CAD build for the part. Positions are in the model's coordinates, mm. A direction names the side the tool comes from. Round coordinates to 2 decimals unless told otherwise and drop trailing zeros. Loops run counter-clockwise (first coordinate to the right, second up) from the corner with the lowest first, then second, coordinate; pieces in that order, holes last. Notation, with made-up numbers: M 54.5,88.25 L 69.5,88.25 A13 ccw 69.5,93.25 Z; hole C 49,-23 d7. An arc over 180 degrees is marked long. Use a Markdown table: item, result. Add a question column.
(1) Band-saw the part on C-C, the plane x = 0. Write the cut outline in (y, z), and give its area (3 significant figures).
(2) Band-saw the part on B-B, the plane z = -22.5. Write the cut outline in (x, y), and give its area (4 significant figures).
(3) Band-saw the part on A-A, the plane y = 42. Write the cut outline in (x, z), and give its area (3 significant figures).
(4) Band-saw the part on D-D, the plane z = 37. Write the cut outline in (x, y), and give its area (3 significant figures).
(5) Flat gauge pins, fed straight in: P1, Ø1, axis at x = -55.5, z = -54, coming from the -Y side; P2, Ø10, axis at x = 7, z = 30.5, coming from the +Y side; P3, Ø2.5, axis at x = 34.5, y = 20.4, coming from the -Z side; P4, Ø6, axis at x = 43.5, y = 22.5, coming from the -Z side. Where does each tip first touch, or does it go through?
(6) Which spindle directions (+Z, -Z, +X, -X, +Y, -Y) get a long thin tool onto all of the face, cutting with end or side? Do faces 5 (the face through (6, 18, 52.5)), 6 (the face through (47.263, 26.302, 53.486)). Say none if no direction does.
(7) Two-plate mould, pull along Z, no slides. Class faces 1 (the face through (-79.398, 21.336, -53.514)), 2 (the face through (6, 18, 54.5)), 3 (the face through (9, 14, -54.5)), 4 (the face through (-2, 0, -1)): released by +Z, released by -Z, zero draft, split by the parting line, or undercut.
(8) Wall check: L1, parallel to Z at x = 75, y = 5; L2, parallel to Y at x = 43, z = 53; L3, parallel to Y at x = 43.5, z = -53.2. Give the ranges that are in metal, low to high.
from build123d import *

# Parameters (mm, degrees)
SKETCH3_W                       = 250
SKETCH3_H                       = 105
BASE_FLANGE1_DEPTH              = 2
EDGE_FLANGE1_STRIP_W            = 10
EDGE_FLANGE1_STRIP_H            = 2
EDGE_FLANGE1_STRIP_CUT_DEPTH    = 217
EDGE_FLANGE1_RELIEF_W           = 11
EDGE_FLANGE1_RELIEF_H           = 1
EDGE_FLANGE1_RELIEF_CUT_DEPTH   = 2
EDGE_FLANGE1_STRIP_2_W          = 10
EDGE_FLANGE1_STRIP_2_H          = 2
EDGE_FLANGE1_STRIP_CUT_2_DEPTH  = 217
EDGE_FLANGE1_RELIEF_2_W         = 11
EDGE_FLANGE1_RELIEF_2_H         = 1
EDGE_FLANGE1_RELIEF_CUT_2_DEPTH = 2
EDGE_FLANGE1_DEPTH              = 217
EDGE_FLANGE1_START              = 2
EDGE_FLANGE1_PROFILE_R          = 5
EDGE_FLANGE1_FLAT_DEPTH         = 2
EDGE_FLANGE1_BEND_DEPTH         = 217
EDGE_FLANGE1_PROFILE_2_R        = 5
EDGE_FLANGE1_FLAT_2_DEPTH       = 2
CUT_EXTRUDE2_START              = -78.75
CUT_EXTRUDE2_DEPTH              = 46.25
CUT_EXTRUDE1_DEPTH              = 144.597527834
CUT_EXTRUDE1_DEPTH_BACK         = 144.597527834
SKETCH14_R                      = 1
SKETCH14_R_2                    = 7


# Read off the part's stored shape, not the designer's step: Cut-Extrude2
# Sheet-metal steps are written as plain solids
with BuildPart() as part:
    # Sketch3 → Base-Flange1 (new body)
    with BuildSketch(Plane(origin=(0, 0, 0), x_dir=(1, 0, 0), z_dir=(0, 1, 0))):
        Rectangle(SKETCH3_W, SKETCH3_H)
    extrude(amount=-BASE_FLANGE1_DEPTH)

    # Edge-Flange1 strip (across the edge) → Edge-Flange1 strip cut (cut)
    with BuildSketch(Plane(origin=(-125, 0, 52.5), x_dir=(0, 0, -1), z_dir=(1, 0, 0))):
        with Locations((-4, -1)):
            Rectangle(EDGE_FLANGE1_STRIP_W, EDGE_FLANGE1_STRIP_H)
    extrude(amount=EDGE_FLANGE1_STRIP_CUT_DEPTH, mode=Mode.SUBTRACT)

    # Edge-Flange1 relief (on the sheet) → Edge-Flange1 relief cut (cut)
    with BuildSketch(Plane(origin=(-125, 0, 51.5), x_dir=(0, 0, -1), z_dir=(0, 1, 0))):
        with Locations((-4.5, -217.5)):
            Rectangle(EDGE_FLANGE1_RELIEF_W, EDGE_FLANGE1_RELIEF_H)
    extrude(amount=-EDGE_FLANGE1_RELIEF_CUT_DEPTH, mode=Mode.SUBTRACT)

    # Edge-Flange1 strip 2 (across the edge) → Edge-Flange1 strip cut 2 (cut)
    with BuildSketch(Plane(origin=(92, 0, -52.5), x_dir=(0, 0, 1), z_dir=(-1, 0, 0))):
        with Locations((-4, -1)):
            Rectangle(EDGE_FLANGE1_STRIP_2_W, EDGE_FLANGE1_STRIP_2_H)
    extrude(amount=EDGE_FLANGE1_STRIP_CUT_2_DEPTH, mode=Mode.SUBTRACT)

    # Edge-Flange1 relief 2 (on the sheet) → Edge-Flange1 relief cut 2 (cut)
    with BuildSketch(Plane(origin=(92, 0, -51.5), x_dir=(0, 0, 1), z_dir=(0, 1, 0))):
        with Locations((-4.5, 0.5)):
            Rectangle(EDGE_FLANGE1_RELIEF_2_W, EDGE_FLANGE1_RELIEF_2_H)
    extrude(amount=-EDGE_FLANGE1_RELIEF_CUT_2_DEPTH, mode=Mode.SUBTRACT)

    # Edge-Flange1 bend section (across the edge) → Edge-Flange1 (add)
    with BuildSketch(Plane(origin=(-125, 0, 52.5), x_dir=(0, 0, -1), z_dir=(1, 0, 0))):
        with BuildLine():
            Line((-2, 1), (0, 1))
            ThreePointArc((0, 1), (0.292893219, 0.292893219), (1, 0))
            Line((1, 0), (1, -2))
            ThreePointArc((1, -2), (-1.121320344, -1.121320344), (-2, 1))
        make_face()
    extrude(amount=EDGE_FLANGE1_DEPTH)

    # Edge-Flange1 profile (on flange) → Edge-Flange1 flat (add)
    with BuildSketch(Plane.XY.offset(52.5).offset(EDGE_FLANGE1_START)):
        with BuildLine():
            Line((-125, 9.993471807), (-125, 1))
            Line((-125, 1), (92, 1))
            Line((92, 1), (92, 33))
            Line((92, 33), (14.696938457, 33))
            ThreePointArc((14.696938457, 33), (0, 45), (-14.696938457, 33))
            Line((-14.696938457, 33), (-32.5, 33))
            Line((-32.5, 33), (-125, 9.993471807))
        make_face()
        with Locations((0, 30)):
            Circle(EDGE_FLANGE1_PROFILE_R, mode=Mode.SUBTRACT)
    extrude(amount=-EDGE_FLANGE1_FLAT_DEPTH)

    # Edge-Flange1 bend section 2 (across the edge) → Edge-Flange1 bend (add)
    with BuildSketch(Plane(origin=(92, 0, -52.5), x_dir=(0, 0, 1), z_dir=(-1, 0, 0))):
        with BuildLine():
            Line((-2, 1), (0, 1))
            ThreePointArc((0, 1), (0.292893219, 0.292893219), (1, 0))
            Line((1, 0), (1, -2))
            ThreePointArc((1, -2), (-1.121320344, -1.121320344), (-2, 1))
        make_face()
    extrude(amount=EDGE_FLANGE1_BEND_DEPTH)

    # Edge-Flange1 profile 2 (on flange) → Edge-Flange1 flat 2 (add)
    with BuildSketch(Plane(origin=(0, 0, -52.5), x_dir=(-1, 0, 0), z_dir=(0, 0, -1)).offset(EDGE_FLANGE1_START)):
        with BuildLine():
            Line((-92, 33), (-92, 1))
            Line((-92, 1), (125, 1))
            Line((125, 1), (125, 9.993471807))
            Line((125, 9.993471807), (32.5, 33))
            Line((32.5, 33), (14.696938457, 33))
            ThreePointArc((14.696938457, 33), (0, 45), (-14.696938457, 33))
            Line((-14.696938457, 33), (-92, 33))
        make_face()
        with Locations((0, 30)):
            Circle(EDGE_FLANGE1_PROFILE_2_R, mode=Mode.SUBTRACT)
    extrude(amount=-EDGE_FLANGE1_FLAT_2_DEPTH)

    # Cut-Extrude2 outline → Cut-Extrude2 (cut)
    with BuildSketch(Plane.YZ.offset(CUT_EXTRUDE2_START)):
        with BuildLine():
            Line((0, -54.328427125), (0.666666667, -52.442809042))
            ThreePointArc((0.666666667, -52.442809042), (0.183503419, -52.077350269), (0, -51.5))
            Line((0, -51.5), (0, -17.5))
            Line((0, -17.5), (-2, -17.5))
            Line((-2, -17.5), (-2, -51.5))
            ThreePointArc((-2, -51.5), (-1.449489743, -53.232050808), (0, -54.328427125))
        make_face()
    extrude(amount=CUT_EXTRUDE2_DEPTH, mode=Mode.SUBTRACT)

    # Sketch14 → Cut-Extrude1 (cut, two sides: drawn at the far end of the back side and taken through both)
    with BuildSketch(Plane.XY.offset(-CUT_EXTRUDE1_DEPTH_BACK)):
        with BuildLine():
            Line((-46.5, 14.125), (-65.166666667, 14.125))
            ThreePointArc((-65.166666667, 14.125), (-67.291666667, 12), (-65.166666667, 9.875))
            Line((-65.166666667, 9.875), (-46.5, 9.875))
            ThreePointArc((-46.5, 9.875), (-44.375, 12), (-46.5, 14.125))
        make_face()
        with BuildLine():
            Line((-57.900010285, 4.380710415), (-51.653085966, 4.380710415))
            ThreePointArc((-51.653085966, 4.380710415), (-50.153085966, 5.880710415), (-51.653085966, 7.380710415))
            Line((-51.653085966, 7.380710415), (-57.900010285, 7.380710415))
            ThreePointArc((-57.900010285, 7.380710415), (-59.400010285, 5.880710415), (-57.900010285, 4.380710415))
        make_face()
        with BuildLine():
            Line((-51.653085966, 4.380710415), (-39.233343618, 4.380710415))
            ThreePointArc((-39.233343618, 4.380710415), (-37.733343618, 5.880710415), (-39.233343618, 7.380710415))
            Line((-39.233343618, 7.380710415), (-51.653085966, 7.380710415))
            ThreePointArc((-51.653085966, 7.380710415), (-50.153085966, 5.880710415), (-51.653085966, 4.380710415))
        make_face()
        with BuildLine():
            Line((-70.319752633, 4.380710415), (-57.900010285, 4.380710415))
            ThreePointArc((-57.900010285, 4.380710415), (-59.400010285, 5.880710415), (-57.900010285, 7.380710415))
            Line((-57.900010285, 7.380710415), (-70.319752633, 7.380710415))
            ThreePointArc((-70.319752633, 7.380710415), (-71.819752633, 5.880710415), (-70.319752633, 4.380710415))
        make_face()
        with BuildLine():
            Line((-72.433323049, 16.619289585), (-60.0135807, 16.619289585))
            ThreePointArc((-60.0135807, 16.619289585), (-61.5135807, 18.119289585), (-60.0135807, 19.619289585))
            Line((-60.0135807, 19.619289585), (-72.433323049, 19.619289585))
            ThreePointArc((-72.433323049, 19.619289585), (-73.933323049, 18.119289585), (-72.433323049, 16.619289585))
        make_face()
        with BuildLine():
            Line((-60.0135807, 16.619289585), (-53.766656382, 16.619289585))
            ThreePointArc((-53.766656382, 16.619289585), (-52.266656382, 18.119289585), (-53.766656382, 19.619289585))
            Line((-53.766656382, 19.619289585), (-60.0135807, 19.619289585))
            ThreePointArc((-60.0135807, 19.619289585), (-61.5135807, 18.119289585), (-60.0135807, 16.619289585))
        make_face()
        with BuildLine():
            ThreePointArc((-53.766656382, 19.619289585), (-52.266656382, 18.119289585), (-53.766656382, 16.619289585))
            Line((-53.766656382, 16.619289585), (-41.346914034, 16.619289585))
            ThreePointArc((-41.346914034, 16.619289585), (-39.846914034, 18.119289585), (-41.346914034, 19.619289585))
            Line((-41.346914034, 19.619289585), (-53.766656382, 19.619289585))
        make_face()
        with Locations((43.5, 11.4)):
            Circle(SKETCH14_R)
        with Locations((52.5, 20.4)):
            Circle(SKETCH14_R)
        with Locations((43.5, 20.4)):
            Circle(SKETCH14_R_2)
        with Locations((34.5, 20.4)):
            Circle(SKETCH14_R)
        with Locations((43.5, 29.4)):
            Circle(SKETCH14_R)
    extrude(amount=CUT_EXTRUDE1_DEPTH + CUT_EXTRUDE1_DEPTH_BACK, mode=Mode.SUBTRACT)


solid = part.part
Return value:
| question | item | result |
|---|---|---|
| 1 | outline | M -2,-51.5 A3 ccw 1,-54.5 L 25,-54.5 L 25,-52.5 L 1,-52.5 A1 cw 0,-51.5 L 0,51.5 A1 cw 1,52.5 L 25,52.5 L 25,54.5 L 1,54.5 A3 ccw -2,51.5 Z; M 35,-54.5 L 45,-54.5 L 45,-52.5 L 35,-52.5 Z; M 35,52.5 L 45,52.5 L 45,54.5 L 35,54.5 Z |
| 1 | area | 355 mm^2 |
| 2 | outline | M -125,-2 L -78.75,-2 L -78.75,0 L -125,0 Z; M -32.5,-2 L 125,-2 L 125,0 L -32.5,0 Z |
| 2 | area | 407.5 mm^2 |
| 3 | outline | M -9,-54.5 L 9,-54.5 L 9,-52.5 L -9,-52.5 Z; M -9,52.5 L 9,52.5 L 9,54.5 L -9,54.5 Z |
| 3 | area | 72.0 mm^2 |
| 4 | outline | M -125,-2 L 125,-2 L 125,0 L -125,0 Z |
| 4 | area | 500 mm^2 |
| 5 | P1 | y = 0 |
| 5 | P2 | y = 0 |
| 5 | P3 | z = -54.5 |
| 5 | P4 | through |
| 6 | face 5 | +X, -X, +Y |
| 6 | face 6 | +Z, -Z |
| 7 | face 1 | zero draft |
| 7 | face 2 | released by +Z |
| 7 | face 3 | released by -Z |
| 7 | face 4 | undercut |
| 8 | L1 | -54.5 to -52.5, 52.5 to 54.5 |
| 8 | L2 | -1.6 to 10.53, 12.27 to 13.42, 27.38 to 28.53, 30.27 to 33 |
| 8 | L3 | -1.47 to 10.4, 12.4 to 13.4, 27.4 to 28.4, 30.4 to 33 |
